Model file for the job. Use its own axes, mm. A direction names the side the tool comes from. Round coordinates to 2 decimals unless told otherwise and drop trailing zeros. Order: outer loops, then holes, each group sorted by start corner. A loop starts at its lowest first (then second) coordinate and runs counter-clockwise, first axis right, second up. Notation, with made-up numbers: (-14, 68) - (45, 68) arc R17 ccw to (45, 73) - close; hole circle Ø5 at (57, 31). An arc over 180 degrees is marked (long way). Use one line per item in the form item = value.
from build123d import *

# Parameters (mm, degrees)
F0_R         = 7.5
F0_R_2       = 2.5
F1_DEPTH     = 200
F2_R         = 1.5
F3_DEPTH     = 25
F4_W         = 255.6320726871
F4_H         = 34.7503256053
F5_DEPTH     = 25
F6_W         = 10
F6_H         = 5
F6_H_2       = 4.8793365061
F7_DEPTH     = 4
F8_R         = 1.5
F9_DEPTH     = 7.501
F11_DEPTH    = 20
F12_T2_ANGLE = 359.64
F12_T4_ANGLE = 359.64


# Not quite as in the source:
# - a fillet or chamfer that OpenCascade refuses, or shapes differently, is made with other operations: its cross-section is extruded or revolved along the edge and cut away or added


with BuildPart() as f1:
    # F0 (on Front) → F1 (new body)
    with BuildSketch(Plane.XZ):
        Circle(F0_R)
        Circle(F0_R_2, mode=Mode.SUBTRACT)
    extrude(amount=-F1_DEPTH)

    # F2 (on face) → F3 (cut)
    with BuildSketch(Plane.XZ):
        with Locations((5, 0)):
            Circle(F2_R)
        with Locations((-5, 0)):
            Circle(F2_R)
    extrude(amount=-F3_DEPTH, mode=Mode.SUBTRACT)

    # F4 (on Right) → F5 (cut)
    with BuildSketch(Plane.YZ):
        with Locations((127.8160363436, -0.9753750637)):
            Rectangle(F4_W, F4_H)
    extrude(amount=F5_DEPTH, mode=Mode.SUBTRACT)

    # F6 (on face) → F7 (join)
    with BuildSketch(Plane.YZ):
        with BuildLine():
            ThreePointArc((10, 7.5), (5, 12.5), (0, 7.5))
            Line((0, 7.5), (10, 7.5))
        make_face()
        with Locations((5, 5)):
            Rectangle(F6_W, F6_H)
        with BuildLine():
            Line((190, 7.5), (200, 7.5))
            ThreePointArc((200, 7.5), (195, 12.5), (190, 7.5))
        make_face()
        with Locations((195, 5)):
            Rectangle(F6_W, F6_H)
        with BuildLine():
            ThreePointArc((190, -7.5), (195, -12.5), (200, -7.5))
            Line((200, -7.5), (190, -7.5))
        make_face()
        with Locations((195, -5.0603317469)):
            Rectangle(F6_W, F6_H_2)
        with BuildLine():
            Line((10, -7.5), (0, -7.5))
            ThreePointArc((0, -7.5), (5, -12.5), (10, -7.5))
        make_face()
        with Locations((5, -5.0603317469)):
            Rectangle(F6_W, F6_H_2)
    extrude(amount=-F7_DEPTH)

    # F8 (on face) → F9 (cut, through all)
    with BuildSketch(Plane.YZ):
        with Locations((5, 10)):
            Circle(F8_R)
        with Locations((5, -10)):
            Circle(F8_R)
        with Locations((195, 10)):
            Circle(F8_R)
        with Locations((195, -10)):
            Circle(F8_R)
    extrude(amount=-F9_DEPTH, mode=Mode.SUBTRACT)

    # F10 (on face) → F11 (join)
    with BuildSketch(Plane(origin=(0, 200, 0), x_dir=(-1, 0, 0), z_dir=(0, 1, 0))):
        with BuildLine():
            ThreePointArc((0, 2), (2, 0), (0, -2))
            Line((0, -2), (0, -2.5))
            ThreePointArc((0, -2.5), (2.5, 0), (0, 2.5))
            Line((0, 2.5), (0, 2))
        make_face()
    extrude(amount=-F11_DEPTH)

    # F12: fillet of radius 2 on 2 edges, made by hand

    # F12_s1 → F12_t2 (revolve, cut)
    with BuildSketch(Plane(origin=(0, 0, 0), x_dir=(0, 1, 0), z_dir=(0.0031415875, 0, -0.9999950652))):
        with BuildLine():
            ThreePointArc((180, 2.5), (180.6157688743, 2.1291713066), (181.3228756555, 2))
            Line((181.3228756555, 2), (180, 2))
            Line((180, 2), (180, 2.5))
        make_face()
    revolve(axis=Axis((0, 180, 0), (0, -1, 0)), revolution_arc=F12_T2_ANGLE, mode=Mode.SUBTRACT)

    # F12_s3 → F12_t4 (revolve, cut)
    with BuildSketch(Plane(origin=(0, 0, 0), x_dir=(0, 1, 0), z_dir=(0.0031415875, 0, -0.9999950652))):
        with BuildLine():
            ThreePointArc((198, 2), (199.4142135624, 2.5857864376), (200, 4))
            Line((200, 4), (200, 2))
            Line((200, 2), (198, 2))
        make_face()
    revolve(axis=Axis((0, 200, 0), (0, -1, 0)), revolution_arc=F12_T4_ANGLE, mode=Mode.SUBTRACT)


solid = f1.part
(1) Tool access for faces 1 (the face through (-4, 195, 8)), 2 (the face through (-2.5, 88.7, 0.1)), 3 (the face through (-4, 195, -8)): list every direction of +Z, -Z, +X, -X, +Y, -Y with a clear straight run to the whole face (end or side of a thin tool).
Report:
face_1 = +Z, -X, +Y, -Y
face_2 = +X, -Y
face_3 = -Z, -X, +Y, -Y
(2) Pin check, flat tips, straight feed: pin 1 (2 mm diameter, centred on x = -6, y = 119, fed in from +Z); pin 2 (4 mm diameter, centred on x = -1, y = 33, fed in from +Z); pin 3 (3 mm diameter, centred on y = 4.5, z = -10.5, fed in from -X); pin 4 (1 mm diameter, centred on x = -3.5, z = -0.5, fed in from -Y). Stop position of each tip, or through.
Report:
pin_1 = 5.59
pin_2 = 7.5
pin_3 = -4
pin_4 = 0
(3) Slice it at B-B on y = 83. Give the cut face in (x, z).
Report:
outline = (0, -7.5) - (0, -2.5) arc R2.5 cw to (0, 2.5) - (0, 7.5) arc R7.5 ccw to start
(4) Pull direction Z, two halves, no side cores. Call faces 4 (the face through (-7.5, 98.6, 0.16)), 5 (the face through (-2, 190, 0)), 6 (the face through (0, 101, -5)): released by +Z, released by -Z, zero draft, split by the parting line, or undercut.
Report:
face_4 = split by the parting line
face_5 = undercut
face_6 = zero draft
(5) Probe probe 1 along Z at (x, y) = (-2.85, 5); probe 2 along Z at (x, y) = (-2.3, 5); probe 3 along Z at (x, y) = (-1.25, 5). List the from-to ranges inside material, lowest first. Write a range as [from, to].
Report:
probe_1 = [-12.5, -11.5], [-8.5, 8.5], [11.5, 12.5]
probe_2 = [-12.5, -11.5], [-8.5, -0.98], [0.98, 8.5], [11.5, 12.5]
probe_3 = [-12.5, -11.5], [-8.5, -2.17], [2.17, 8.5], [11.5, 12.5]
(6) Slice it at A-A on y = 186.5. Give the cut face in (x, z), then the cut area to 3 significant figures.
Report:
outline = (0, -7.5) - (0, -2) arc R2 cw to (0, 2) - (0, 7.5) arc R7.5 ccw to start
area = 82.1 mm2
